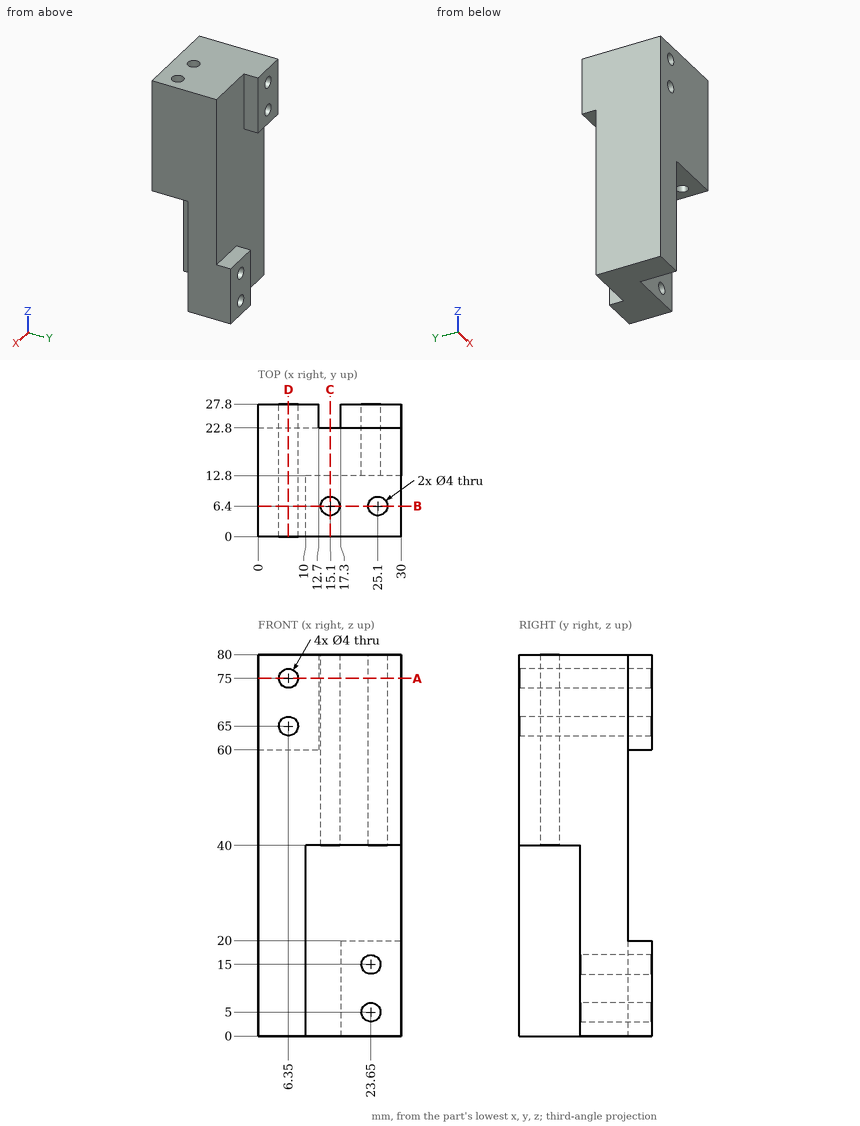
Job drawing, mm, ordinate dimensions from the low corner. One solid piece. Coordinates: 2 decimals unless noted, no trailing zeros. Order: outer loops, then holes, each group sorted by start corner. A loop starts at its lowest first (then second) coordinate and runs counter-clockwise, first axis right, second up. Notation, with made-up numbers: (46, 40) -> (66, 40) arc R25 ccw to (66, 79) -> close; hole circle Ø1 at (31.25, -24.75). An arc over 180 degrees is marked (long way). Answer in a Markdown table with one row per item. Add a question column.
Q1. Drop flat-ended pins along their axis: pin 1 (6 mm diameter, centred on x = 21, z = 28, fed in from -Y); pin 2 (2 mm diameter, centred on x = 20.5, z = 55.5, fed in from +Y); pin 3 (1.5 mm diameter, centred on y = 26, z = 5.5, fed in from -X). Give the stop position or say it passes through.
Q2. Band-saw the part on A-A, the plane z = 75. List the corners of the cut face in (x, y), then the cut area to 3 significant figures.
Q3. Band-saw the part on C-C, the plane x = 15.1. List the corners of the cut face in (y, z), then the cut area to 3 significant figures.
Q4. Band-saw the part on D-D, the plane x = 6.35. List the corners of the cut face in (y, z), then the cut area to 3 significant figures.
Q5. Wall check: line 1 along X through (y, z) = (22, 5); line 2 along Y through (x, z) = (15.1, 60.5); line 3 along X through (y, z) = (9.5, 75). Give the ranges that are in metal, low to high. Write a range as [from, to].
Q6. Band-saw the part on B-B, the plane y = 6.4. List the corners of the cut face in (x, z).
Answers follow:
| question | item | result |
|---|---|---|
| 1 | pin 1 | y = 12.8 |
| 1 | pin 2 | y = 22.8 |
| 1 | pin 3 | x = 17.3 |
| 2 | outline | (0, 0) -> (4.35, 0) -> (4.35, 27.8) -> (0, 27.8) -> close; (8.35, 0) -> (30, 0) -> (30, 22.8) -> (12.7, 22.8) -> (12.7, 27.8) -> (8.35, 27.8) -> close; hole circle Ø4 at (15.1, 6.4); hole circle Ø4 at (25.1, 6.4) |
| 2 | area | 611 mm^2 |
| 3 | outline | (0, 40) -> (4.4, 40) -> (4.4, 80) -> (0, 80) -> close; (8.4, 40) -> (12.8, 40) -> (12.8, 0) -> (22.8, 0) -> (22.8, 80) -> (8.4, 80) -> close |
| 3 | area | 1,150 mm^2 |
| 4 | outline | (0, 0) -> (22.8, 0) -> (22.8, 60) -> (27.8, 60) -> (27.8, 63) -> (0, 63) -> close; (0, 67) -> (27.8, 67) -> (27.8, 73) -> (0, 73) -> close; (0, 77) -> (27.8, 77) -> (27.8, 80) -> (0, 80) -> close |
| 4 | area | 1,700 mm^2 |
| 5 | line 1 | [0, 21.65], [25.65, 30] |
| 5 | line 2 | [0, 4.4], [8.4, 22.8] |
| 5 | line 3 | [0, 4.35], [8.35, 30] |
| 6 | outline | (0, 0) -> (10, 0) -> (10, 40) -> (13.1, 40) -> (13.1, 80) -> (0, 80) -> close; (17.1, 40) -> (23.1, 40) -> (23.1, 80) -> (17.1, 80) -> close; (27.1, 40) -> (30, 40) -> (30, 80) -> (27.1, 80) -> close; hole circle Ø4 at (6.35, 65); hole circle Ø4 at (6.35, 75) |
